```python
from build123d import *

# Parameters (mm, degrees)
SKETCH2_W           = 20
SKETCH2_H           = 20
BOSS_EXTRUDE1_DEPTH = 5
SKETCH3_R           = 2.1
CUT_EXTRUDE1_DEPTH  = 5
FILLET2_R           = 2.5
SKETCH5_R           = 1.6
BOSS_EXTRUDE2_DEPTH = 5
FILLET4_R           = 2.5
SKETCH6_R           = 1.6
CUT_EXTRUDE2_DEPTH  = 10


with BuildPart() as part:
    # Sketch2 → Boss-Extrude1 (new body)
    with BuildSketch(Plane.XY):
        Rectangle(SKETCH2_W, SKETCH2_H)
    extrude(amount=BOSS_EXTRUDE1_DEPTH)

    # Sketch3 → Cut-Extrude1 (cut)
    with BuildSketch(Plane.XY.offset(5)):
        Circle(SKETCH3_R)
    extrude(amount=-CUT_EXTRUDE1_DEPTH, mode=Mode.SUBTRACT)

    # Fillet2
    fillet2_edges = [part.edges().sort_by_distance(p)[0] for p in [
        (10, -10, 2.5),
        (-10, -10, 2.5),
    ]]
    fillet(fillet2_edges, radius=FILLET2_R)

    # Sketch5 → Boss-Extrude2 (add)
    with BuildSketch(Plane(origin=(0, 10, 0), x_dir=(1, 0, 0), z_dir=(0, 1, 0))):
        Polygon((-10, -5), (10, -5), (10, 4.190598923), (6, 6.5), (6, 11.5), (10, 13.809401077), (10, 23), (-10, 23), (-10, 13.809401077), (-6, 11.5), (-6, 6.5), (-10, 4.190598923), align=None)
        with Locations(Location((0, 2.141483503, 0), (0, 0, 270))):
            Circle(SKETCH5_R, mode=Mode.SUBTRACT)
        with Locations(Location((0, 19.641483503, 0), (0, 0, 270))):
            Circle(SKETCH5_R, mode=Mode.SUBTRACT)
    extrude(amount=BOSS_EXTRUDE2_DEPTH)

    # Fillet4
    fillet4_edges = [part.edges().sort_by_distance(p)[0] for p in [
        (-10, 15, 0.404700538),
        (10, 15, 0.404700538),
        (10, 12.5, -23),
        (-10, 12.5, -23),
    ]]
    fillet(fillet4_edges, radius=FILLET4_R)

    # Sketch6 → Cut-Extrude2 (cut)
    with BuildSketch(Plane(origin=(0, 0, 0), x_dir=(-1, 0, 0), z_dir=(0, 0, -1))):
        with Locations((-6, 6)):
            Circle(SKETCH6_R)
        with Locations((6, 6)):
            Circle(SKETCH6_R)
        with Locations((6, -6)):
            Circle(SKETCH6_R)
        with Locations((-6, -6)):
            Circle(SKETCH6_R)
    extrude(amount=-CUT_EXTRUDE2_DEPTH, mode=Mode.SUBTRACT)


solid = part.part
```
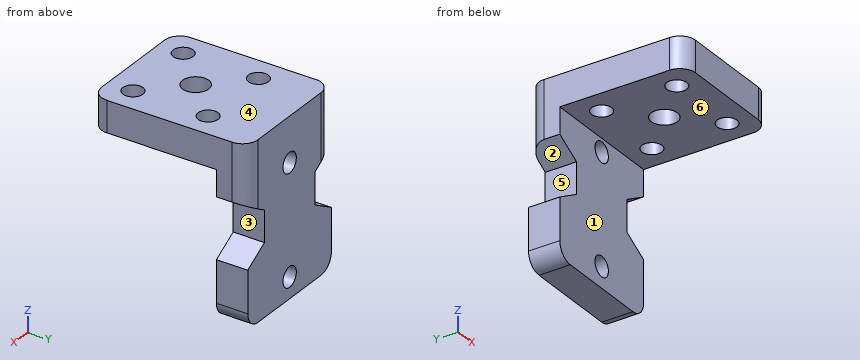
For this review, take the finished solid that the model builds, in its own axes (mm). Face numbers are marked on the shaded views. A direction names the side the tool comes from. Coordinates: 2 decimals unless noted, no trailing zeros. Loops run counter-clockwise (first coordinate to the right, second up) from the corner with the lowest first, then second, coordinate; pieces in that order, holes last.
1. Add section C-C, the plane z = -2. Give the boundary of the cut face in (x, y), then the cut area to 3 significant figures.
2. Add section A-A, the plane x = 0. Give the boundary of the cut face in (y, z), then the cut area to 3 significant figures.
3. For the marked faces 1, 2 and 3, list the 3-axis set-ups (+Z, -Z, +X, -X, +Y, -Y) from which the entire face can be reached by the end or side of a thin tool; tool diameter is ignored.
4. Add section D-D, the plane y = 1. Give the boundary of the cut face in (x, z).
5. Add section B-B, the plane y = -6. Give the boundary of the cut face in (x, z), then the cut area to 3 significant figures.
6. Insertion check: P1, Ø10, axis at x = 4.5, z = -13, coming from the -Y side; P2, Ø2.5, axis at y = 11.5, z = -10, coming from the -X side; P3, Ø4, axis at y = 13, z = -9, coming from the +X side. Each pin has a flat end and moves straight along its axis. Give the tip position at first contact, or say it passes through.
7. For line 1 (Y direction, x = 6, z = 1.55); line 2 (Z direction, x = -8, y = 3); line 3 (Y direction, x = -5.5, z = -9.25), list the stretches that pass through material, from the lowest coordinate up.
8. Mouldability with a two-part tool opening along Z and no side actions: class the marked faces 4, 5 and 6 as +Z half, -Z half, draft (parallel to the pull), parting line (faces both ways), or undercut.
Result:
1. outline: (-10, 10) - (-1.59, 10) - (-1.59, 15) - (-7.5, 15) arc R2.5 ccw to (-10, 12.5) - close; (1.59, 10) - (10, 10) - (10, 12.5) arc R2.5 ccw to (7.5, 15) - (1.59, 15) - close
1. area: 81.4 mm2
2. outline: (-10, 0) - (-2.1, 0) - (-2.1, 5) - (-10, 5) - close; (2.1, 0) - (10, 0) - (10, -0.54) - (15, -0.54) - (15, 5) - (2.1, 5) - close; (10, -23) - (15, -23) - (15, -21.24) - (10, -21.24) - close; (10, -18.04) - (15, -18.04) - (15, -3.74) - (10, -3.74) - close
2. area: 187 mm2
3. face 1: -Z, +X, -X, -Y
3. face 2: -X, +Y, -Y
3. face 3: +X, +Y, -Y
4. outline: (-10, 0) - (-1.85, 0) - (-1.85, 5) - (-10, 5) - close; (1.85, 0) - (10, 0) - (10, 5) - (1.85, 5) - close
5. outline: (-10, 0) - (-7.6, 0) - (-7.6, 5) - (-10, 5) - close; (-4.4, 0) - (4.4, 0) - (4.4, 5) - (-4.4, 5) - close; (7.6, 0) - (10, 0) - (10, 5) - (7.6, 5) - close
5. area: 68.0 mm2
6. P1: stops at y = 10
6. P2: stops at x = -6
6. P3: stops at x = 6
7. line 1: y = -10 to -7.6, -4.4 to 4.4, 7.6 to 15
7. line 2: z = 0 to 5
7. line 3: y = 10 to 15
8. face 4: +Z half
8. face 5: undercut
8. face 6: -Z half
